Could you check a few things on this model? Use its own coordinates, in mm. Coordinates: 2 decimals unless noted, no trailing zeros. Loops run counter-clockwise (first coordinate to the right, second up) from the corner with the lowest first, then second, coordinate; pieces in that order, holes last. Notation, with made-up numbers: (68.5, -9) - (106.5, -9) arc R3 cw to (106.5, -4) - close; hole circle Ø11 at (0, 34.5). An arc over 180 degrees is marked (long way). One line per item, written item: value. Start each with the question number.
(1) If we section it at D-D on y = -117: Write out the boundary of the cut face in (x, z).
(2) If we section it at C-C on x = -114: Write out the boundary of the cut face in (y, z), then the cut area to 3 significant figures.
(3) If we section it at B-B on x = -217.5: Write out the boundary of the cut face in (y, z), then the cut area to 3 significant figures.
(4) I'm going to push flat-ended pins straight in: P1, Ø8.5, axis at x = -72, z = -0.5, coming from the +Y side; P2, Ø2, axis at y = -181, z = -11, coming from the +X side; P3, Ø3, axis at x = -63.5, z = 11.5, coming from the -Y side. Where does each tip first touch, or does it pass through?
(5) If we section it at A-A on y = -175: Write out the boundary of the cut face in (x, z).
(6) If I drill on line 1 along Z through (x, y) = (-246.75, -175); line 2 along Z through (x, y) = (-245, -175); line 3 along Z through (x, y) = (-228, -98.5), over which ranges is the centre line in solid material (lowest first)? Write a range as from..to.
```python
from build123d import *

# Parameters (mm, degrees)
EXTRUSION1_DEPTH        = 12.5
ESQUISSE2_R             = 3
ENL_V_MAT_EXTRU_1_DEPTH = 323.674371464
ESQUISSE3_R             = 2.5
ENL_V_MAT_EXTRU_2_DEPTH = 331.255582845
COQUE1_T                = -4
EXTRUSION2_DEPTH        = 4


with BuildPart() as part:
    # Esquisse1 → Extrusion1 (new, symmetric)
    with BuildSketch(Plane.XY):
        with BuildLine():
            Line((0, 0), (-212.5, 0))
            ThreePointArc((-212.5, 0), (-233.713203436, -8.786796564), (-242.5, -30))
            Line((-242.5, -30), (-242.5, -212.5))
            Line((-242.5, -212.5), (-252.5, -212.5))
            Line((-252.5, -212.5), (-252.5, -30))
            ThreePointArc((-252.5, -30), (-240.784271247, -1.715728753), (-212.5, 10))
            Line((-212.5, 10), (0, 10))
            Line((0, 10), (0, 0))
        make_face()
    extrude(amount=EXTRUSION1_DEPTH, both=True)

    # Esquisse2 → Enlèv. mat.-Extru.1 (cut, through all)
    with BuildSketch(Plane(origin=(-242.5, 0, 0), x_dir=(0, 0, -1), z_dir=(1, 0, 0))):
        with Locations(Location((0, -50, 0), (0, 0, 90))):
            Circle(ESQUISSE2_R)
        with Locations(Location((0, -175, 0), (0, 0, 90))):
            Circle(ESQUISSE2_R)
    extrude(amount=-ENL_V_MAT_EXTRU_1_DEPTH, mode=Mode.SUBTRACT)

    # Esquisse3 → Enlèv. mat.-Extru.2 (cut, through all)
    with BuildSketch(Plane.XZ):
        with Locations((-25, 0)):
            Circle(ESQUISSE3_R)
    extrude(amount=-ENL_V_MAT_EXTRU_2_DEPTH, mode=Mode.SUBTRACT)

    # Coque1
    coque1_openings = [part.faces().sort_by_distance(p)[0] for p in [
        (-252.5, -121.359810516, 0),
        (-240.784271247, -1.715728753, 0),
        (-106.551413319, 10, 0),
    ]]
    offset(amount=COQUE1_T, openings=coque1_openings, kind=Kind.INTERSECTION)

    # Esquisse4 → Extrusion2 (add)
    with BuildSketch(Plane.XY.offset(12.5)):
        with BuildLine():
            Line((-212.5, 0), (0, 0))
            Line((0, 0), (0, -5))
            ThreePointArc((0, -5), (-2.928932188, -12.071067812), (-10, -15))
            Line((-10, -15), (-90.857864376, -15))
            ThreePointArc((-90.857864376, -15), (-94.6846987, -15.761204675), (-97.928932188, -17.928932188))
            Line((-97.928932188, -17.928932188), (-224.571067812, -144.571067812))
            ThreePointArc((-224.571067812, -144.571067812), (-226.738795325, -147.8153013), (-227.5, -151.642135624))
            Line((-227.5, -151.642135624), (-227.5, -202.5))
            ThreePointArc((-227.5, -202.5), (-230.428932188, -209.571067812), (-237.5, -212.5))
            Line((-237.5, -212.5), (-242.5, -212.5))
            Line((-242.5, -212.5), (-242.5, -30))
            ThreePointArc((-242.5, -30), (-233.713203436, -8.786796564), (-212.5, 0))
        make_face()
        with BuildLine():
            Line((-212.5, -15), (-140.355339059, -15))
            ThreePointArc((-140.355339059, -15), (-131.116543734, -21.173165676), (-133.284271247, -32.071067812))
            Line((-133.284271247, -32.071067812), (-210.428932188, -109.215728753))
            ThreePointArc((-210.428932188, -109.215728753), (-221.326834324, -111.383456266), (-227.5, -102.144660941))
            Line((-227.5, -102.144660941), (-227.5, -30))
            ThreePointArc((-227.5, -30), (-223.106601718, -19.393398282), (-212.5, -15))
        make_face(mode=Mode.SUBTRACT)
    extrusion2 = extrude(amount=-EXTRUSION2_DEPTH)

    # Symétrie1: Extrusion2 across plane
    add(extrusion2.mirror(Plane.XY))


solid = part.part
```
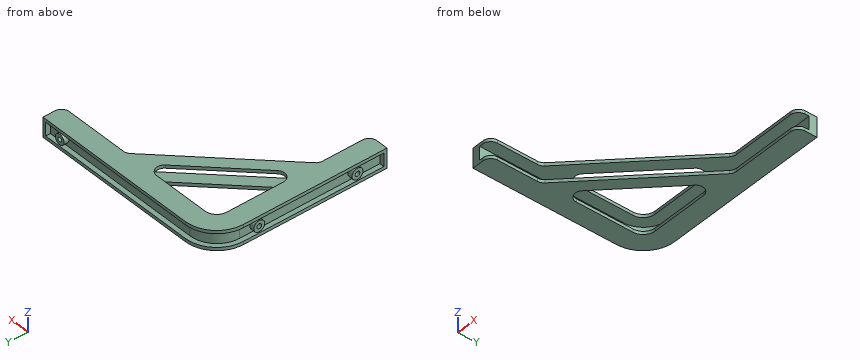
Values:
1. outline: (-252.5, -12.5) - (-197, -12.5) - (-197, -8.5) - (-242.5, -8.5) - (-242.5, 8.5) - (-197, 8.5) - (-197, 12.5) - (-252.5, 12.5) - (-252.5, 8.5) - (-246.5, 8.5) - (-246.5, -8.5) - (-252.5, -8.5) - close
2. outline: (-34, -12.5) - (10, -12.5) - (10, -8.5) - (4, -8.5) - (4, 8.5) - (10, 8.5) - (10, 12.5) - (-34, 12.5) - (-34, 8.5) - (0, 8.5) - (0, -8.5) - (-34, -8.5) - close
2. area: 420 mm2
3. outline: (-137.5, -12.5) - (-112.14, -12.5) - (-112.14, -8.5) - (-137.5, -8.5) - close; (-137.5, 8.5) - (-112.14, 8.5) - (-112.14, 12.5) - (-137.5, 12.5) - close; (-15.86, -12.5) - (9.69, -12.5) - (9.69, -8.5) - (3.63, -8.5) - (3.63, 8.5) - (9.69, 8.5) - (9.69, 12.5) - (-15.86, 12.5) - (-15.86, 8.5) - (-0.42, 8.5) - (-0.42, -8.5) - (-15.86, -8.5) - close
3. area: 476 mm2
4. P1: stops at y = 4
4. P2: stops at x = -227.5
4. P3: stops at y = -15
5. outline: (-252.5, -12.5) - (-227.5, -12.5) - (-227.5, -8.5) - (-242.5, -8.5) - (-242.5, -3) - (-252.5, -3) - (-252.5, -7) - (-246.5, -7) - (-246.5, -8.5) - (-252.5, -8.5) - close; (-252.5, 3) - (-242.5, 3) - (-242.5, 8.5) - (-227.5, 8.5) - (-227.5, 12.5) - (-252.5, 12.5) - (-252.5, 8.5) - (-246.5, 8.5) - (-246.5, 7) - (-252.5, 7) - close
6. line 1: z = -12.5..-8.5, -7..-3, 3..7, 8.5..12.5
6. line 2: z = -12.5..-3, 3..12.5
6. line 3: z = -12.5..-8.5, 8.5..12.5
